Input: part model. Units: mm. Frame: model coordinates. A direction names the side the tool comes from. Coordinates: 2 decimals unless noted, no trailing zeros. Write each loop counter-clockwise with the first axis right and the second up, starting at its lowest first coordinate (ties: lowest second). Pieces come first, ordered by that corner, then holes.
1) Pin query (flat end, axial travel): pin 1 Ø5 at (x, y) = (-6, -9.5) entering from +Z; pin 2 Ø4 at (x, y) = (2.5, 7) entering from -Z. Return the tip coordinate at first contact, or that it passes through.
2) Line query: L1, parallel to X at y = -0.5, z = -330.5 (3 decimals). Output: solid intervals per line, ascending.
3) Draft query along X for faces 3 (the flat face through (9.525, 0, -6)), 4 (the flat face through (0, 12.7, -6)), 5 (the flat face through (-12.7, 0, -6)), 6 (the flat face through (12.7, 0, -6)). Return one class per face: pulls with the +X half, pulls with the -X half, needs draft (parallel to the pull), parting line crosses it, or undercut.
4) Section query A-A (x = -5.5). Output: boundary loops of the cut face in (y, z) (3 decimals), then the cut area to 3 significant figures.
5) Section query C-C (z = 328). Output: boundary loops of the cut face in (x, y) (3 decimals).
6) Set-up query: faces 1 (the flat face through (11, 0, 457.2)), 2 (the flat face through (0, -9.525, -6)). Return all of +Z, -Z, +X, -X, +Y, -Y with unobstructed straight access to the full face (end or side cutting, diameter ignored); none if empty.
Autodesk Inventor part; units mm, degrees
ref_plane "YZ Plane" through (0, 0, 0) normal (1, 0, 0) x (0, 1, 0)
ref_plane "XZ Plane" through (0, 0, 0) normal (0, 1, 0) x (-1, 0, 0)
ref_plane "XY Plane" through (0, 0, 0) normal (0, 0, 1) x (1, 0, 0)
sketch "Sketch1" plane through (0, 0, 0) normal (0, 0, 1) x (1, 0, 0)
  line L0 (-17.78, 0) -> (17.78, 0)
  line L1 (0, -17.78) -> (0, 17.78)
  line L2 (-12.7, 12.7) -> (12.7, 12.7)
  line L3 (12.7, 12.7) -> (12.7, -12.7)
  line L4 (12.7, -12.7) -> (-12.7, -12.7)
  line L5 (-12.7, -12.7) -> (-12.7, 12.7)
  line L6 (9.525, 9.525) -> (-9.525, 9.525)
  line L7 (-9.525, 9.525) -> (-9.525, -9.525)
  line L8 (-9.525, -9.525) -> (9.525, -9.525)
  line L9 (9.525, -9.525) -> (9.525, 9.525)
  point P0 (0, 0)
  point P1 (-12.7, 0)
  point P2 (0, 12.7)
  dimension "d0" = 25.4
  dimension "d1" = 3.175
extrude "Extrusion1" add sketch "Sketch1" along normal mid plane 914.4 contours L5 L2 L1 L6 L7 L0 | L0 L7 L8 L1 L4 L5 | L1 L8 L9 L0 L3 L4 | L2 L3 L0 L9 L6 L1
properties part number "tubing_template_0.125" material "Aluminum-6061"
Answer:
1. pin 1: stops at z = 457.2
1. pin 2: passes through
2. L1: x = -12.7 to -9.525, 9.525 to 12.7
3. face 3: undercut
3. face 4: needs draft
3. face 5: pulls with the -X half
3. face 6: pulls with the +X half
4. outline: (-12.7, -457.2) - (-9.525, -457.2) - (-9.525, 457.2) - (-12.7, 457.2) - close; (9.525, -457.2) - (12.7, -457.2) - (12.7, 457.2) - (9.525, 457.2) - close
4. area: 5,810 mm2
5. outline: (-12.7, -12.7) - (12.7, -12.7) - (12.7, 12.7) - (-12.7, 12.7) - close; hole (-9.525, -9.525) - (9.525, -9.525) - (9.525, 9.525) - (-9.525, 9.525) - close
6. face 1: +Z, +X, -X, +Y, -Y
6. face 2: +Z, -Z
